The model under review builds one solid part; all positions refer to its coordinate system, in mm. Face numbers are marked on the shaded views. A direction names the side the tool comes from. Round coordinates to 2 decimals unless told otherwise and drop trailing zeros. Order: outer loops, then holes, each group sorted by start corner. A loop starts at its lowest first (then second) coordinate and runs counter-clockwise, first axis right, second up. Notation, with made-up numbers: M 50.5,-15.75 L 99.5,-15.75 A27 ccw 99.5,13.25 Z; hole C 16.5,84.25 d11. An arc over 180 degrees is marked long. Use a Markdown table: item, result. Add a question column.
1. Consider section A-A on y = 57.15. State the section outline as (x, z) points (3 decimals), then the cut area to 3 significant figures.
2. To check wall thickness, follow probe 1 along Y at (x, z) = (-0.45, 12.7); probe 2 along Y at (x, z) = (-16.65, 0.3) (3 decimals); probe 3 along Z at (x, y) = (-14.5, 16.5). State the ranges of each line that lie inside material, in increasing order.
3. For the marked faces 1 and 2, list the 3-axis set-ups (+Z, -Z, +X, -X, +Y, -Y) from which the entire face can be reached by the end or side of a thin tool; tool diameter is ignored.
4. Consider section D-D on y = 35.45. State the section outline as (x, z) points (3 decimals).
5. Consider section C-C on x = -6.35. State the section outline as (y, z) points (3 decimals).
6. Insertion check: P1, Ø3, axis at x = -4.5, y = 34.5, coming from the +Z side; P2, Ø9, axis at y = 24.5, z = 8.5, coming from the -X side; P3, Ø6, axis at x = -8, z = 3, coming from the -Y side. Each pin has a flat end and moves straight along its axis. Give the tip position at first contact, or say it passes through.
7. Consider section B-B on z = 12. State the section outline as (x, y) points, then the cut area to 3 significant figures.
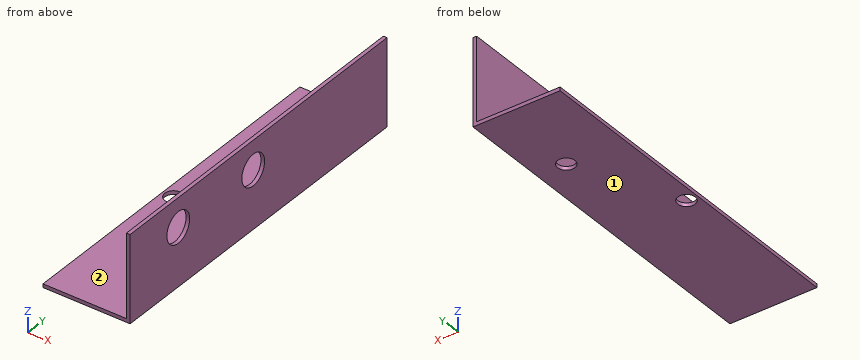
Autodesk Inventor part; units mm, degrees
ref_plane "YZ Plane" through (0, 0, 0) normal (1, 0, 0) x (0, 1, 0)
ref_plane "XZ Plane" through (0, 0, 0) normal (0, 1, 0) x (-1, 0, 0)
ref_plane "XY Plane" through (0, 0, 0) normal (0, 0, 1) x (1, 0, 0)
sketch "Sketch1" plane through (0, 0, 0) normal (0, 1, 0) x (-1, 0, 0)
  line L0 (0, 0) -> (0, 19.05)
  line L1 (0, 19.05) -> (0.7937, 19.05)
  line L2 (0.7937, 19.05) -> (0.7938, 0.7937)
  line L3 (0.7938, 0.7937) -> (19.05, 0.7937)
  line L4 (19.05, 0.7937) -> (19.05, 0)
  line L5 (19.05, 0) -> (0, 0)
  dimension "d0" = 19.05
  dimension "d1" = 0.7937
extrude "Extrusion1" add sketch "Sketch1" along normal blind 76.2
sketch "Sketch2" plane through (0, 0, 19.05) normal (1, 0, 0) x (0, 0, -1)
  line L0 (19.05, 0) -> (19.05, 76.2)
  line L1 (6.35, 36.5125) -> (6.35, 14.2875) construction
  circle A0 centre (6.35, 36.5125) radius 3.3782
  circle A1 centre (6.35, 14.2875) radius 3.3782
  line L2 (19.05, 0) -> (0, 0)
  dimension "d4" = 22.225
  dimension "d5" = 6.7564
  dimension "d16" = 12.7
  dimension "d17" = 14.2875
extrude "Extrusion2" cut sketch "Sketch2" against normal through all
sketch "Sketch3" plane through (0, 0, 0) normal (0, 0, -1) x (-1, 0, 0)
  line L0 (0, 76.2) -> (19.05, 76.2)
  line L1 (0, 0) -> (0, 76.2)
  line L2 (16.65, 57.15) -> (6.35, 57.15) construction
  line L3 (6.35, 57.15) -> (6.35, 35.45) construction
  line L4 (6.35, 35.45) -> (16.65, 35.45) construction
  line L5 (16.65, 35.45) -> (16.65, 57.15) construction
  circle A0 centre (16.65, 35.45) radius 1.905
  circle A1 centre (6.35, 57.15) radius 1.905
  dimension "d9" = 3.81
  dimension "d10" = 21.7
  dimension "d11" = 10.3
  dimension "d12" = 19.05
  dimension "d13" = 6.35
extrude "Extrusion3" cut sketch "Sketch3" against normal through all
properties part number "Limit Switch Bracket Shooter Front Right Corner" material "Aluminum 6061"
Answer block:
| question | item | result |
|---|---|---|
| 1 | outline | M -19.05,0 L -8.255,0 L -8.255,0.794 L -19.05,0.794 Z; M -4.445,0 L 0,0 L 0,19.05 L -0.794,19.05 L -0.794,0.794 L -4.445,0.794 Z |
| 1 | area | 26.6 mm^2 |
| 2 | probe 1 | 0 to 10.91, 17.67 to 33.13, 39.89 to 76.2 |
| 2 | probe 2 | 0 to 33.545, 37.355 to 76.2 |
| 2 | probe 3 | 0 to 0.79 |
| 3 | face 1 | -Z, +X, -X, +Y, -Y |
| 3 | face 2 | +Z, -X, +Y, -Y |
| 4 | outline | M -19.05,0 L -18.555,0 L -18.555,0.794 L -19.05,0.794 Z; M -14.745,0 L 0,0 L 0,9.493 L -0.794,9.493 L -0.794,0.794 L -14.745,0.794 Z; M -0.794,15.907 L 0,15.907 L 0,19.05 L -0.794,19.05 Z |
| 5 | outline | M 0,0 L 55.245,0 L 55.245,0.794 L 0,0.794 Z; M 59.055,0 L 76.2,0 L 76.2,0.794 L 59.055,0.794 Z |
| 6 | P1 | z = 0.79 |
| 6 | P2 | x = -0.79 |
| 6 | P3 | y = 0 |
| 7 | outline | M -0.79,0 L 0,0 L 0,10.98 L -0.79,10.98 Z; M -0.79,17.59 L 0,17.59 L 0,33.21 L -0.79,33.21 Z; M -0.79,39.82 L 0,39.82 L 0,76.2 L -0.79,76.2 Z |
| 7 | area | 50.0 mm^2 |
